Read the model definition and answer for the solid it produces. Units are mm, in the model's axes. Face numbers are marked on the shaded views. A direction names the side the tool comes from. Give positions to 0.01 mm unless a question says otherwise; leave off trailing zeros. Loops run counter-clockwise (first coordinate to the right, second up) from the corner with the lowest first, then second, coordinate; pieces in that order, holes last.
(1) Find section C-C, the plane y = 1. Write down the section's boundary in (x, z).
(2) Find section A-A, the plane z = 0. Write down the section's boundary in (x, y), then the cut area to 3 significant figures.
(3) Each of these flat-tipped pins is pushed along its axis until it touches: P1, Ø0.6, axis at x = 0.5, y = 0.5, coming from the +Z side; P2, Ø2, axis at x = 1.5, y = 2.5, coming from the -Z side; P3, Ø0.6, axis at x = 0, y = 0.5, coming from the +Z side. Where does it stop, or does it pass through?
(4) Find section B-B, the plane y = 8.25. Write down the section's boundary in (x, z), then the cut area to 3 significant figures.
(5) Straight lines are drawn through the part: probe 1 along X at (y, z) = (7.5, 0); probe 2 along Y at (x, z) = (0.7, 0.2); probe 3 along Y at (x, z) = (-1.8, -0.5). For each, find the intervals that lie inside material, in ascending order.
(6) Which of the six approach directions +Z, -Z, +X, -X, +Y, -Y give full straight-line access (tool end or side, diameter ignored) to the marked faces 1 and 2?
```python
from build123d import *

# Parameters (mm, degrees)
SKETCH1_R           = 1.25
BOSS_EXTRUDE1_DEPTH = 10
CUT_EXTRUDE1_DEPTH  = 0.5


with BuildPart() as part:
    # Sketch1 → Boss-Extrude1 (new body)
    with BuildSketch(Plane(origin=(0, 0, 0), x_dir=(1, 0, 0), z_dir=(0, 1, 0))):
        with Locations(Location((0, 0, 0), (0, 0, 270))):
            Circle(SKETCH1_R)
    extrude(amount=BOSS_EXTRUDE1_DEPTH)

    # Sketch2 → Revolve1 (revolve)
    with BuildSketch(Plane(origin=(0, 0, 0), x_dir=(0, 0, -1), z_dir=(1, 0, 0)), mode=Mode.PRIVATE) as revolve1_sk:
        Polygon((0, 0), (0, 1.5), (-1.25, 1.5), (-2.35, 0.1), (-2.35, 0), align=None)
    revolve(revolve1_sk.sketch.rotate(Axis((0, -0.5, 0), (0, 1, 0)), 180), axis=Axis((0, -0.5, 0), (0, 1, 0)))

    # Sketch3 → Cut-Extrude1 (cut)
    with BuildSketch(Plane.XZ):
        Polygon((-1.5, -0.25), (-0.25, -0.25), (-0.25, -1.5), (0.25, -1.5), (0.25, -0.25), (1.5, -0.25), (1.5, 0.25), (0.25, 0.25), (0.25, 1.5), (-0.25, 1.5), (-0.25, 0.25), (-1.5, 0.25), align=None)
    extrude(amount=-CUT_EXTRUDE1_DEPTH, mode=Mode.SUBTRACT)


solid = part.part
```
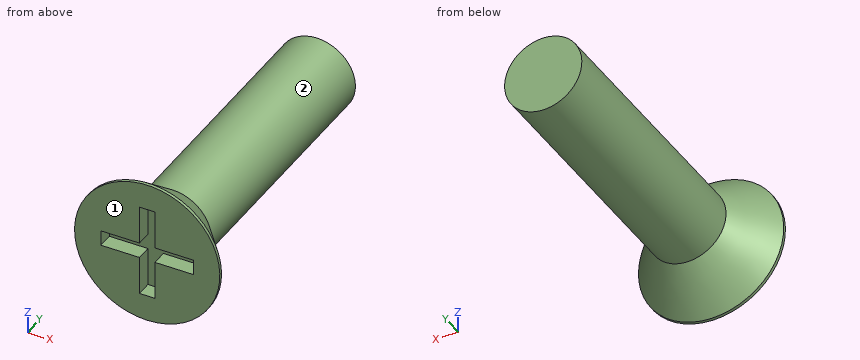
Entries:
1. outline: circle Ø3.29 at (0, 0)
2. outline: (-2.35, 0) - (-1.5, 0) - (-1.5, 0.5) - (1.5, 0.5) - (1.5, 0) - (2.35, 0) - (2.35, 0.1) - (1.25, 1.5) - (1.25, 10) - (-1.25, 10) - (-1.25, 1.5) - (-2.35, 0.1) - close
2. area: 25.3 mm2
3. P1: stops at z = 2.22
3. P2: stops at z = -1.15
3. P3: stops at z = 2.27
4. outline: circle Ø2.5 at (0, 0)
4. area: 4.91 mm2
5. probe 1: x = -1.25 to 1.25
5. probe 2: y = 0.5 to 10
5. probe 3: y = 0 to 0.71
6. face 1: +Z, -Z, +X, -X, -Y
6. face 2: +Y
